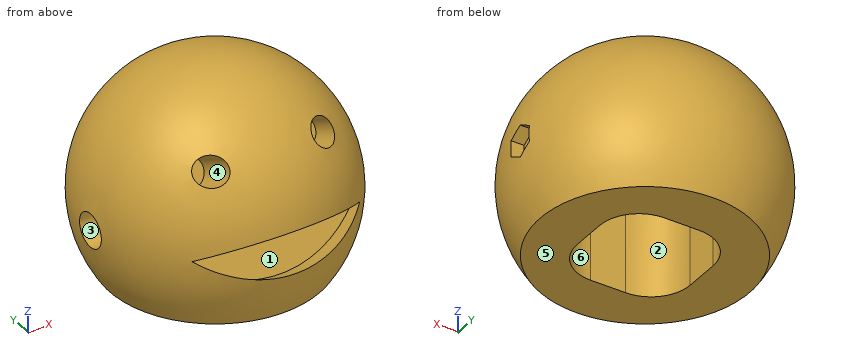
```python
from build123d import *

# Parameters (mm, degrees)
F2_W      = 90.5019028811
F2_H      = 17.7580579312
F3_DEPTH  = 40
F5_DEPTH  = 20.25
F6_R      = 3
F7_DEPTH  = 50
F8_R      = 14
F11_R     = 5
F12_DEPTH = 40
F15_R     = 6
F16_DEPTH = 8
F18_DEPTH = 5


with BuildPart() as f1:
    # F0 (on Top) → F1 (revolve)
    with BuildSketch(Plane.XY):
        with BuildLine():
            Line((0, -45), (0, 45))
            ThreePointArc((0, 45), (-45, 0), (0, -45))
        make_face()
    revolve(axis=Axis((0, 2.1741483361, 0), (0, 1, 0)))

    # F2 (on Front) → F3 (cut, symmetric)
    with BuildSketch(Plane.XZ):
        with Locations((5.2887741476, -33.8790289656)):
            Rectangle(F2_W, F2_H)
    extrude(amount=F3_DEPTH, both=True, mode=Mode.SUBTRACT)

    # F4 (on Front) → F5 (cut, symmetric)
    with BuildSketch(Plane.XZ):
        with BuildLine():
            Line((-20.25, 5), (-20.25, -54.200690622))
            Line((-20.25, -54.200690622), (20.25, -54.200690622))
            Line((20.25, -54.200690622), (20.25, 5))
            ThreePointArc((20.25, 5), (0, -15.25), (-20.25, 5))
        make_face()
        with BuildLine():
            ThreePointArc((20.25, 5), (0, 25.25), (-20.25, 5))
            Line((-20.25, 5), (20.25, 5))
        make_face()
        with BuildLine():
            Line((20.25, 5), (-20.25, 5))
            ThreePointArc((-20.25, 5), (0, -15.25), (20.25, 5))
        make_face()
    extrude(amount=F5_DEPTH, both=True, mode=Mode.SUBTRACT)

    # F6 (on Right) → F7 (cut, symmetric)
    with BuildSketch(Plane.YZ):
        Circle(F6_R)
    extrude(amount=F7_DEPTH, both=True, mode=Mode.SUBTRACT)

    # F8
    f8_edges = [f1.edges().sort_by_distance(p)[0] for p in [
        (-20.25, -20.25, -10),
        (-20.25, 20.25, -10),
        (20.25, -20.25, -10),
        (20.25, 20.25, -10),
        (0, -20.25, 25.25),
        (0, 20.25, 25.25),
    ]]
    fillet(f8_edges, radius=F8_R)

    # F11 (on face) → F12 (cut)
    with BuildSketch(Plane(origin=(0, -56.3237066798, 32.5185072133), x_dir=(1, 0, 0), z_dir=(0, -0.8660254038, 0.5))):
        with BuildLine():
            Line((30, -15), (-30, -15))
            ThreePointArc((-30, -15), (0, -28.2363828336), (30, -15))
        make_face()
        with Locations((-20, 10)):
            Circle(F11_R)
        with Locations((20, 10)):
            Circle(F11_R)
    extrude(amount=-F12_DEPTH, mode=Mode.SUBTRACT)

    # F15 (on offset) → F16 (cut)
    with BuildSketch(Plane.YZ.offset(-45)):
        Circle(F15_R)
    extrude(amount=F16_DEPTH, mode=Mode.SUBTRACT)

    # F17 (on offset) → F18 (cut)
    with BuildSketch(Plane.YZ.offset(45)):
        Polygon((5, -2.8867513459), (5, 2.8867513459), (0, 5.7735026919), (-5, 2.8867513459), (-5, -2.8867513459), (0, -5.7735026919), align=None)
    extrude(amount=-F18_DEPTH, mode=Mode.SUBTRACT)


solid = f1.part
```
Can you work these out from the model? Positions are in its coordinate system, mm. Face numbers are marked on the shaded views. A direction names the side the tool comes from. Round coordinates to 2 decimals unless told otherwise and drop trailing zeros. Order: outer loops, then holes, each group sorted by start corner. A loop starts at its lowest first (then second) coordinate and runs counter-clockwise, first axis right, second up. Notation, with made-up numbers: (-39.5, 75.25) -> (-10.5, 75.25) arc R21 ccw to (-10.5, 100.25) -> close; hole circle Ø10 at (62.5, -18.5). An arc over 180 degrees is marked (long way). Return JSON: item names as keys, results as strings. Group by question number.
1. If we section it at B-B, the plane x = 35.5: Write out the boundary of the cut face in (y, z).
2. If we section it at C-C, the plane z = 18.5: Count the separate pieces of the cut face and the enclosed holes in it, then the cut area to 3 significant figures.
3. I need wall thicknesses on line 1 (X direction, y = -17.5, z = 23); line 2 (Y direction, x = 7, z = -14.5); line 3 (Y direction, x = -41.5, z = 0). Which ranges of each line are inside material? Lowest first, please. Write a range as [from, to].
4. If we section it at D-D, the plane y = 36: Write out the boundary of the cut face in (x, z), then the cut area to 3 significant figures.
5. Which directions (+Z, -Z, +X, -X, +Y, -Y) give clear straight access to the entire face, cutting with the end or side of a thin tool? Please do the marked faces 1, 2 and 3.
6. Will these pins go through, and if not, where does the flat tip stop? pin 1 (14 mm diameter, centred on y = 3, z = -9, fed in from +X); pin 2 (3 mm diameter, centred on x = 27, z = -10, fed in from -Y); pin 3 (10 mm diameter, centred on y = -1, z = -16.5, fed in from -X).
7. If we section it at A-A, the plane z = -15: Write out the boundary of the cut face in (x, y), then the cut area to 3 significant figures.
8. We'd pull the mould along Z, two halves only. Please class the marked faces 4, 5 and 6: released by +Z, released by -Z, zero draft, split by the parting line, or undercut.
Output values:
{
 "1": {"outline": "(-11.82, -25) -> (11.82, -25) arc R27.65 ccw (long way) to start; hole circle Ø6 at (0, 0)"},
 "2": {"separate pieces": "1", "enclosed holes": "3", "area": "4,290 mm²"},
 "3": {"line 1": "[-34.49, -24.86], [-15.14, 15.14], [24.86, 34.49]", "line 2": "[-42.02, -20.23], [20.23, 42.02]", "line 3": "[-17.4, -6], [6, 17.4]"},
 "4": {"outline": "(-10.2, -25) -> (10.2, -25) arc R27 ccw (long way) to start", "area": "2,260 mm²"},
 "5": {"face 1": "none", "face 2": "-Z", "face 3": "-X"},
 "6": {"pin 1": "x = 44.72", "pin 2": "y = -35.78", "pin 3": "x = -43.5"},
 "7": {"outline": "circle Ø84.85 at (0, 0); hole (-20.25, -6.25) arc R14 ccw to (-6.25, -20.25) -> (6.25, -20.25) arc R14 ccw to (20.25, -6.25) -> (20.25, 6.25) arc R14 ccw to (6.25, 20.25) -> (-6.25, 20.25) arc R14 ccw to (-20.25, 6.25) -> close", "area": "4,180 mm²"},
 "8": {"face 4": "undercut", "face 5": "released by -Z", "face 6": "zero draft"}
}
